```python
from build123d import *

# Parameters (mm, degrees)
CROQUIS1_R              = 4
CROQUIS1_R_2            = 50
SALIENTE_EXTRUIR1_DEPTH = 2
ESCALA1_SCALE           = 0.5


with BuildPart() as part:
    # Croquis1 → Saliente-Extruir1 (new body)
    with BuildSketch(Plane.XY):
        with BuildLine():
            Line((63.995308988, 8.006149239), (59.46344738, 8.006149239))
            ThreePointArc((59.46344738, 8.006149239), (-60, 0), (59.46344738, -8.006149239))
            Line((59.46344738, -8.006149239), (63.995308988, -8.006149239))
            Line((63.995308988, -8.006149239), (63.995308988, 8.006149239))
        make_face()
        with BuildLine():
            Line((63, -7), (59.590267662, -7))
            ThreePointArc((59.590267662, -7), (60, 0), (59.590267662, 7))
            Line((59.590267662, 7), (63, 7))
            Line((63, 7), (63, -7))
        make_face(mode=Mode.SUBTRACT)
        with Locations((0, 55)):
            Circle(CROQUIS1_R, mode=Mode.SUBTRACT)
        with Locations((55, 0)):
            Circle(CROQUIS1_R, mode=Mode.SUBTRACT)
        with Locations((0, -55)):
            Circle(CROQUIS1_R, mode=Mode.SUBTRACT)
        with Locations((-55, 0)):
            Circle(CROQUIS1_R, mode=Mode.SUBTRACT)
        Circle(CROQUIS1_R_2, mode=Mode.SUBTRACT)
    extrude(amount=SALIENTE_EXTRUIR1_DEPTH)


with BuildPart() as part_1:
    # Escala1: scaled about (0.43933496, 0, 1)
    add(part.part.scale(ESCALA1_SCALE).moved(Location((0.21966748, 0, 0.5))))


solid = part_1.part
```
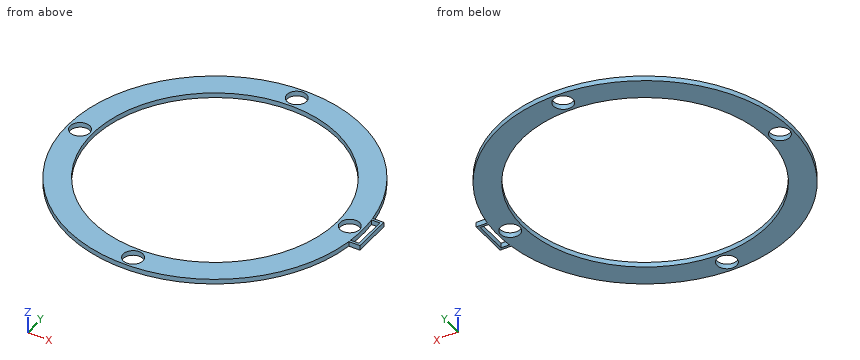
Build history of the part. All positions in model axes, mm. Round coordinates to 2 decimals unless told otherwise and drop trailing zeros. Order: outer loops, then holes, each group sorted by start corner. A loop starts at its lowest first (then second) coordinate and runs counter-clockwise, first axis right, second up. Notation, with made-up numbers: (-2.75, 11.25) - (10.25, 11.25) arc R4 ccw to (10.25, 16.25) - close; hole circle Ø6 at (-2, 47.25). An arc over 180 degrees is marked (long way). Use a Markdown table: item, result.
1) Saw through at B-B on y = 0. Write the cut outline in (x, z), and give its area (3 significant figures).
Recorded:
| item | result |
|---|---|
| outline | (-29.78, 0.5) - (-29.28, 0.5) - (-29.28, 1.5) - (-29.78, 1.5) - close; (-25.28, 0.5) - (-24.78, 0.5) - (-24.78, 1.5) - (-25.28, 1.5) - close; (25.22, 0.5) - (25.72, 0.5) - (25.72, 1.5) - (25.22, 1.5) - close; (29.72, 0.5) - (30.22, 0.5) - (30.22, 1.5) - (29.72, 1.5) - close; (31.72, 0.5) - (32.22, 0.5) - (32.22, 1.5) - (31.72, 1.5) - close |
| area | 2.50 mm² |
2) Saw through at D-D on x = 16. Write the cut outline in (y, z), and give its area (3 significant figures).
Recorded:
| item | result |
|---|---|
| outline | (-25.51, 0.5) - (-19.39, 0.5) - (-19.39, 1.5) - (-25.51, 1.5) - close; (19.39, 0.5) - (25.51, 0.5) - (25.51, 1.5) - (19.39, 1.5) - close |
| area | 12.2 mm² |
3) Flat gauge pins, fed straight in: pin 1 Ø6.5 at (x, y) = (-27.28, 0) entering from +Z; pin 2 Ø0.5 at (x, z) = (30.5, 1) entering from -Y. Where does each tip first touch, or does it go through?
Recorded:
| item | result |
|---|---|
| pin 1 | stops at z = 1.5 |
| pin 2 | stops at y = -4 |
4) Wall check: L1, parallel to X at y = 3, z = 0.8; L2, parallel to Y at x = 12, z = 1.35; L3, parallel to Y at x = -2.5, z = 0.7. Give the ranges that are in metal, low to high.
Recorded:
| item | result |
|---|---|
| L1 | x = -29.63 to -24.6, 25.04 to 30.07, 31.72 to 32.22 |
| L2 | y = -27.59 to -22.05, 22.05 to 27.59 |
| L3 | y = -29.88 to -24.85, 24.85 to 29.88 |
5) Saw through at A-A on z = 0.95. Write the cut outline in (x, y).
Recorded:
| item | result |
|---|---|
| outline | (29.95, -4) - (32.22, -4) - (32.22, 4) - (29.95, 4) arc R30 ccw (long way) to start; hole circle Ø4 at (-27.28, 0); hole circle Ø50 at (0.22, 0); hole circle Ø4 at (0.22, -27.5); hole circle Ø4 at (0.22, 27.5); hole circle Ø4 at (27.72, 0); hole (30.01, -3.5) - (31.72, -3.5) - (31.72, 3.5) - (30.01, 3.5) arc R30 cw to start |
6) Saw through at C-C on x = 1.5. Write the cut outline in (y, z).
Recorded:
| item | result |
|---|---|
| outline | (-29.97, 0.5) - (-29.04, 0.5) - (-29.04, 1.5) - (-29.97, 1.5) - close; (-25.96, 0.5) - (-24.97, 0.5) - (-24.97, 1.5) - (-25.96, 1.5) - close; (24.97, 0.5) - (25.96, 0.5) - (25.96, 1.5) - (24.97, 1.5) - close; (29.04, 0.5) - (29.97, 0.5) - (29.97, 1.5) - (29.04, 1.5) - close |
